Autodesk Inventor part; units mm, degrees
ref_plane "YZ Plane" through (0, 0, 0) normal (1, 0, 0) x (0, 1, 0)
ref_plane "XZ Plane" through (0, 0, 0) normal (0, 1, 0) x (-1, 0, 0)
ref_plane "XY Plane" through (0, 0, 0) normal (0, 0, 1) x (1, 0, 0)
sketch "Sketch1" plane through (0, 0, 0) normal (0, 0, 1) x (1, 0, 0)
  line L0 (-10, 10) -> (10, 10)
  line L1 (10, 10) -> (10, -10)
  line L2 (10, -10) -> (-10, -10)
  line L3 (-10, -10) -> (-10, 10)
  point P0 (0, 0)
  dimension "d0" = 20
  dimension "d1" = 10
  dimension "d2" = 10
  dimension "d3" = 10
extrude "Extrusion1" add sketch "Sketch1" along normal blind 10
sketch "Sketch2" plane through (0, 0, 0) normal (0, 0, -1) x (-1, 0, 0)
  circle A0 centre (0, -4) radius 3
  line L0 (0, -4) -> (0, 0) construction
  circle A1 centre (-7, -5.5) radius 1.6
  circle A2 centre (7, -5.5) radius 1.6
  dimension "d6" = 6
  dimension "d7" = 4
  dimension "d8" = 3.2
  dimension "d9" = 7
  dimension "d10" = 5.5
sketch "Sketch3" plane through (10, -10, 0) normal (1, 0, 0) x (0, 0, -1)
  circle A0 centre (-5, 15.5) radius 3.025
  point P0 (0, 10)
  point P1 (0, 0)
  dimension "d11" = 6.05
  dimension "d12" = 5
  dimension "d13" = 15.5
extrude "Extrusion2" cut sketch "Sketch3" against normal blind 20
extrude "Extrusion3" cut sketch "Sketch2" against normal blind 10
properties part number "ENDER 3 HEATBLOCK" material "Aluminum 6061, Welded"
For this review, take the finished solid that the model builds, in its own axes (mm). Coordinates: 2 decimals unless noted, no trailing zeros. Order: outer loops, then holes, each group sorted by start corner. A loop starts at its lowest first (then second) coordinate and runs counter-clockwise, first axis right, second up. Notation, with made-up numbers: (89, 61) -> (128, 61) arc R22 cw to (128, 89) -> close; hole circle Ø2 at (-7, 61). An arc over 180 degrees is marked (long way). Return JSON: item names as keys, results as strings.
1. The part is to be moulded in two halves that separate along Y. For faces 1 (the flat face through (0, 10, 5)), 2 (the cylindrical face through (0.14, 2.547, 5.656)), 3 (the flat face through (0, 0, 10)), say which applies: +Y half, -Y half, draft (parallel to the pull), parting line (faces both ways), or undercut.
Answer block:
{"face 1": "+Y half", "face 2": "undercut", "face 3": "draft"}
2. For line 1 (Y direction, x = 0, z = 7); line 2 (Y direction, x = -7.25, z = 3); line 3 (Y direction, x = 0, z = 9.5), list the stretches that pass through material, from the lowest coordinate up. Write a range as from..to.
Answer block:
{"line 1": "-10..-7, -1..3.23, 7.77..10", "line 2": "-10..-7.08, -3.92..3.23, 7.77..10", "line 3": "-10..-7, -1..10"}
3. We need section C-C on y = -5.5. Write out the cut boundary in (x, z).
Answer block:
{"outline": "(-10, 0) -> (-8.6, 0) -> (-8.6, 10) -> (-10, 10) -> close; (-5.4, 0) -> (-2.6, 0) -> (-2.6, 10) -> (-5.4, 10) -> close; (2.6, 0) -> (5.4, 0) -> (5.4, 10) -> (2.6, 10) -> close; (8.6, 0) -> (10, 0) -> (10, 10) -> (8.6, 10) -> close"}
4. We need section B-B on z = 5. Write out the cut boundary in (x, y) (3 decimals).
Answer block:
{"outline": "(-10, -10) -> (10, -10) -> (10, 2.475) -> (-10, 2.475) -> close; (-10, 8.525) -> (10, 8.525) -> (10, 10) -> (-10, 10) -> close; hole circle Ø3.2 at (-7, -5.5); hole circle Ø6 at (0, -4); hole circle Ø3.2 at (7, -5.5)"}
5. We need section A-A on x = 7. Write out the cut boundary in (y, z) (3 decimals), and give its area (3 significant figures).
Answer block:
{"outline": "(-10, 0) -> (-7.1, 0) -> (-7.1, 10) -> (-10, 10) -> close; (-3.9, 0) -> (10, 0) -> (10, 10) -> (-3.9, 10) -> close; hole circle Ø6.05 at (5.5, 5)", "area": "139 mm²"}
6. We need section D-D on x = -5. Write out the cut boundary in (y, z) (3 decimals), and give its area (3 significant figures).
Answer block:
{"outline": "(-10, 0) -> (10, 0) -> (10, 10) -> (-10, 10) -> close; hole circle Ø6.05 at (5.5, 5)", "area": "171 mm²"}
